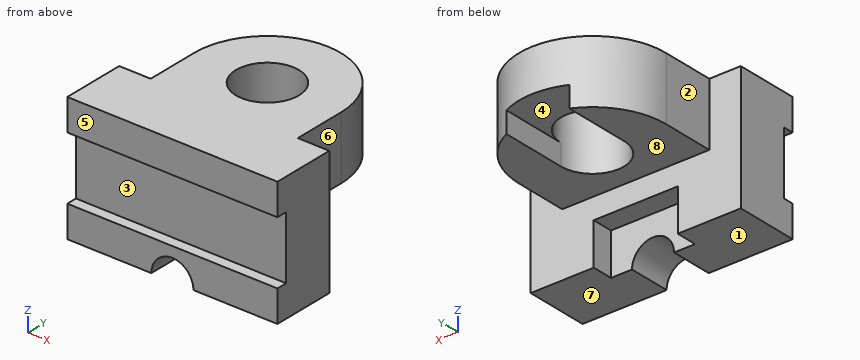
from build123d import *

# Parameters (mm, degrees)
SKETCH1_W           = 40
SKETCH1_H           = 10
BOSS_EXTRUDE1_DEPTH = 60
SKETCH1_3_R         = 15
BOSS_EXTRUDE2_DEPTH = 30
CUT_EXTRUDE1_START  = -40
SKETCH1_4_W         = 40
SKETCH1_4_H         = 10
CUT_EXTRUDE1_DEPTH  = 69.282039139
SKETCH2_W           = 30
SKETCH2_H           = 10
CUT_EXTRUDE2_DEPTH  = 139.654246239
CUT_EXTRUDE3_START  = -10
CUT_EXTRUDE3_DEPTH  = 10
SKETCH4_R           = 10
CUT_EXTRUDE4_DEPTH  = 105.880884817


with BuildPart() as part:
    # Sketch1 → Boss-Extrude1 (new body)
    with BuildSketch(Plane.XY):
        Polygon((-50, 15), (-50, -15), (50, -15), (50, 15), (35, 15), (20, 15), (20, 5), (-20, 5), (-20, 15), (-35, 15), align=None)
        with Locations((0, 10)):
            Rectangle(SKETCH1_W, SKETCH1_H)
    extrude(amount=-BOSS_EXTRUDE1_DEPTH)

    # Sketch1_3 → Boss-Extrude2 (add)
    with BuildSketch(Plane.XY):
        with BuildLine():
            Line((-35, 40), (-35, 15))
            Line((-35, 15), (-20, 15))
            Line((-20, 15), (20, 15))
            Line((20, 15), (35, 15))
            Line((35, 15), (35, 40))
            ThreePointArc((35, 40), (0, 75), (-35, 40))
        make_face()
        with Locations((0, 40)):
            Circle(SKETCH1_3_R, mode=Mode.SUBTRACT)
    extrude(amount=-BOSS_EXTRUDE2_DEPTH)

    # Sketch1_4 → Cut-Extrude1 (cut, through all)
    with BuildSketch(Plane.XY.offset(CUT_EXTRUDE1_START)):
        with Locations((0, 10)):
            Rectangle(SKETCH1_4_W, SKETCH1_4_H)
    extrude(amount=-CUT_EXTRUDE1_DEPTH, mode=Mode.SUBTRACT)

    # Sketch2 → Cut-Extrude2 (cut, through all)
    with BuildSketch(Plane(origin=(50, 0, 0), x_dir=(0, 0, -1), z_dir=(1, 0, 0))):
        with Locations((30, -15)):
            Rectangle(SKETCH2_W, SKETCH2_H)
    extrude(amount=-CUT_EXTRUDE2_DEPTH, mode=Mode.SUBTRACT)

    # Sketch3 → Cut-Extrude3 (cut)
    with BuildSketch(Plane(origin=(0, 0, -30), x_dir=(-1, 0, 0), z_dir=(0, 0, -1)).offset(CUT_EXTRUDE3_START)):
        with BuildLine():
            Line((15, 40), (15, 85.033892836))
            Line((15, 85.033892836), (-15, 85.033892836))
            Line((-15, 85.033892836), (-15, 40))
            ThreePointArc((-15, 40), (0, 25), (15, 40))
        make_face()
    extrude(amount=CUT_EXTRUDE3_DEPTH, mode=Mode.SUBTRACT)

    # Sketch4 → Cut-Extrude4 (cut, through all)
    with BuildSketch(Plane(origin=(0, 5, 0), x_dir=(1, 0, 0), z_dir=(0, 1, 0))):
        with Locations((0, 60)):
            Circle(SKETCH4_R)
    extrude(amount=-CUT_EXTRUDE4_DEPTH, mode=Mode.SUBTRACT)


solid = part.part
Can you work these out from the model? Positions are in its coordinate system, mm. Face numbers are marked on the shaded views. A direction names the side the tool comes from. Coordinates: 2 decimals unless noted, no trailing zeros. Loops run counter-clockwise (first coordinate to the right, second up) from the corner with the lowest first, then second, coordinate; pieces in that order, holes last. Notation, with made-up numbers: (76, -17.5) - (117, -17.5) arc R27 ccw to (117, -0.5) - close; hole circle Ø6 at (45.25, -28). An arc over 180 degrees is marked (long way). Put each result on its own line as item: value. Start each with the question number.
Item 1: Suppose I cut it at A-A (x = 0). Please give me the cut outline in (y, z).
Item 2: Which directions (+Z, -Z, +X, -X, +Y, -Y) give clear straight access to the entire face, cutting with the end or side of a thin tool? Please do the marked faces 4, 5, 6, 7 and 8.
Item 3: For pin 1 (6 mm diameter, centred on y = 29.5, z = -35.5, fed in from +X); pin 2 (4 mm diameter, centred on x = -6, y = -11.5, fed in from -Z); pin 3 (5 mm diameter, centred on y = 63, z = -24, fed in from +X); pin 4 (16 mm diameter, centred on x = -9, z = -49, fed in from +Y), each with a flat end and sliding along its axis, tell me the tip position at first contact or that it passes through.
Item 4: Suppose I cut it at B-B (y = 44.5). Please give me the cut outline in (x, z).
Item 5: If we mould it in two halves opening along Z, with no side actions, what happens to the marked faces 1, 2 and 3? For each: +Z half, -Z half, draft (parallel to the pull), parting line (faces both ways), or undercut.
Item 6: If I drill on line 1 along Y through (x, z) = (0, -16); line 2 along Y through (x, z) = (0, -6.5); line 3 along X through (y, z) = (40, -16), over which ranges is the centre line in solid material (lowest first)?
Item 7: Suppose I cut it at D-D (x = -30). Please give me the cut outline in (y, z).
Item 8: Suppose I cut it at C-C (z = -53.5). Please give me the cut outline in (x, y), and give its area (3 significant figures).
Here are the results:
1. outline: (-15, -50) - (5, -50) - (5, -40) - (15, -40) - (15, -30) - (25, -30) - (25, 0) - (-15, 0) - (-15, -15) - (-10, -15) - (-10, -45) - (-15, -45) - close; (55, -20) - (75, -20) - (75, 0) - (55, 0) - close
2. face 4: -Z, +Y
2. face 5: +Z, -Z, +X, -X, -Y
2. face 6: +Z, -Z, +X, +Y
2. face 7: -Z, +X, -X, +Y, -Y
2. face 8: -Z, +X, -X, +Y
3. pin 1: through
3. pin 2: z = -54
3. pin 3: x = 28.37
3. pin 4: y = 5
4. outline: (-34.71, -30) - (-15, -30) - (-15, -20) - (-14.31, -20) - (-14.31, 0) - (-34.71, 0) - close; (14.31, -20) - (15, -20) - (15, -30) - (34.71, -30) - (34.71, 0) - (14.31, 0) - close
5. face 1: -Z half
5. face 2: draft
5. face 3: undercut
6. line 1: -10 to 25, 55 to 75
6. line 2: -15 to 25, 55 to 75
6. line 3: -35 to -15, 15 to 35
7. outline: (-15, -60) - (15, -60) - (15, -30) - (58.03, -30) - (58.03, 0) - (-15, 0) - (-15, -15) - (-10, -15) - (-10, -45) - (-15, -45) - close
8. outline: (-50, -15) - (-7.6, -15) - (-7.6, 5) - (-20, 5) - (-20, 15) - (-50, 15) - close; (7.6, -15) - (50, -15) - (50, 15) - (20, 15) - (20, 5) - (7.6, 5) - close
8. area: 2,300 mm²
